Can you work these out from the model? Positions are in its coordinate system, mm. Face numbers are marked on the shaded views. Round coordinates to 2 decimals unless told otherwise and drop trailing zeros. Loops run counter-clockwise (first coordinate to the right, second up) from the corner with the lowest first, then second, coordinate; pieces in that order, holes last. Notation, with made-up numbers: M 64.25,51 L 111.25,51 A22 cw 111.25,76 Z; hole C -1,-13.5 d11. An arc over 180 degrees is marked long. Return JSON: item names as keys, results as strings.
Autodesk Inventor part; units mm, degrees
ref_plane "YZ Plane" through (0, 0, 0) normal (1, 0, 0) x (0, 1, 0)
ref_plane "XZ Plane" through (0, 0, 0) normal (0, 1, 0) x (-1, 0, 0)
ref_plane "XY Plane" through (0, 0, 0) normal (0, 0, 1) x (1, 0, 0)
sketch "Szkic1" plane through (0, 0, 0) normal (0, 0, 1) x (1, 0, 0)
  circle A0 centre (0, 0) radius 11
  line L0 (-17.5, -17.5) -> (17.5, -17.5)
  line L1 (17.5, -17.5) -> (17.5, 17.5)
  line L2 (17.5, 17.5) -> (-17.5, 17.5)
  line L3 (-17.5, 17.5) -> (-17.5, -17.5)
  line L4 (-17.5, -17.5) -> (17.5, 17.5) construction
  line L5 (17.5, -17.5) -> (-17.5, 17.5) construction
  dimension "d0" = 22
  dimension "d1" = 35
extrude "Wyciągnięcie proste1" add sketch "Szkic1" along normal blind 12
sketch "Szkic2" plane through (0, 0, 0) normal (1, 0, 0) x (0, 1, 0)
  line L0 (-11, 12) -> (11, 12)
  line L1 (11, 0) -> (-11, 0)
  line L2 (-11, 0) -> (-11, 12)
  line L3 (-11, 10.6) -> (-11.5, 10.6)
  line L4 (-11.5, 10.6) -> (-11.5, 9.5)
  line L5 (-11.5, 9.5) -> (-11, 9.5)
  line L6 (-11, 9.5) -> (-11, 10.6)
  line L7 (11, 0) -> (11, 12) construction
  line L8 (11, 6) -> (-11, 6) construction
  line L9 (-11, 2.5) -> (-11.5, 2.5)
  line L10 (-11.5, 2.5) -> (-11.5, 1.4)
  line L11 (-11.5, 1.4) -> (-11, 1.4)
  line L12 (-11, 1.4) -> (-11, 2.5)
  line L13 (0, 0) -> (0, 12) construction
  dimension "d4" = 1.1
  dimension "d5" = 0.5
  dimension "d8" = 7
revolve "Obrót1" cut sketch "Szkic2" angle 360 about axis through (0, 0, 0) along (0, 0, 1)
sketch "Szkic3" plane through (-17.5, -17.5, 0) normal (0, -1, 0) x (1, 0, 0)
  line L0 (0, 0) -> (35, 0)
  line L1 (35, 0) -> (35, 12)
  line L2 (0, 12) -> (35, 12)
  line L3 (0, 0) -> (0, 12)
  line L4 (35, 6) -> (0, 6) construction
  line L5 (0, 12) -> (35, 12) construction
  line L6 (17.5, 12) -> (17.5, 0) construction
  point P0 (31.5, 6)
  point P1 (3.5, 6)
  dimension "d9" = 28
hole "Otwór1" at (14, -17.5, 6) at (-14, -17.5, 6) direction (0, 1, 0) diameter 4 end through all
properties part number "bearing"
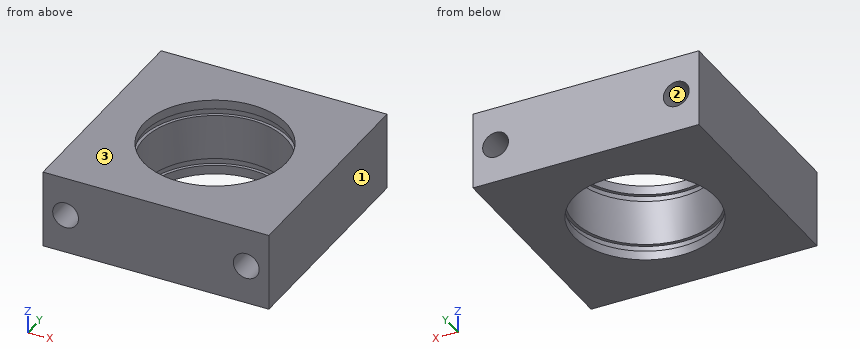
Q1. Suppose I cut it at D-D, the plane y = 12.5. Please give me the cut outline in (x, z), plus the area to 3 significant figures.
Results:
{"outline": "M -17.5,0 L 17.5,0 L 17.5,12 L -17.5,12 Z; hole C -14,6 d4; hole C 14,6 d4", "area": "395 mm2"}
Q2. Suppose I cut it at B-B, the plane z = 6. Please give me the cut outline in (x, y).
Results:
{"outline": "M -17.5,-17.5 L -16,-17.5 L -16,17.5 L -17.5,17.5 Z; M -12,-17.5 L 12,-17.5 L 12,17.5 L -12,17.5 Z; M 16,-17.5 L 17.5,-17.5 L 17.5,17.5 L 16,17.5 Z; hole C 0,0 d22"}
Q3. I'm going to push a flat-ended pin straight in: pin 1 Ø11.5 at (x, y) = (-1, -2) entering from -Z. Where does the tip first touch, or does it pass through?
Results:
{"pin 1": "passes through"}
Q4. Suppose I cut it at A-A, the plane y = 0. Please give me the cut outline in (x, z), plus the area to 3 significant figures.
Results:
{"outline": "M -17.5,0 L -11,0 L -11,1.4 L -11.5,1.4 L -11.5,2.5 L -11,2.5 L -11,9.5 L -11.5,9.5 L -11.5,10.6 L -11,10.6 L -11,12 L -17.5,12 Z; M 11,0 L 17.5,0 L 17.5,12 L 11,12 L 11,10.6 L 11.5,10.6 L 11.5,9.5 L 11,9.5 L 11,2.5 L 11.5,2.5 L 11.5,1.4 L 11,1.4 Z; hole C -14,6 d4; hole C 14,6 d4", "area": "129 mm2"}
Q5. If I drill on line 1 along Z through (x, y) = (14, 3); line 2 along X through (y, z) = (0, 10.95); line 3 along X through (y, z) = (15.5, 5.5), over which ranges is the centre line in solid material (lowest first)?
Results:
{"line 1": "z = 0 to 4, 8 to 12", "line 2": "x = -17.5 to -11, 11 to 17.5", "line 3": "x = -17.5 to -15.94, -12.06 to 12.06, 15.94 to 17.5"}
Q6. Thinking about a two-plate mould opening in X: for the marked faces 1, 2 and 3, which applies, pulls with the +X half, pulls with the -X half, needs draft (parallel to the pull), parting line crosses it, or undercut?
Results:
{"face 1": "pulls with the +X half", "face 2": "undercut", "face 3": "needs draft"}
Q7. Suppose I cut it at C-C, the plane x = -14. Please give me the cut outline in (y, z).
Results:
{"outline": "M -17.5,0 L 17.5,0 L 17.5,4 L -17.5,4 Z; M -17.5,8 L 17.5,8 L 17.5,12 L -17.5,12 Z"}
